```python
from build123d import *

# Parameters (mm, degrees)
F1_DEPTH       = 50.8
F3_DEPTH       = 1066.8
F5_DEPTH       = 26.67
F7_DEPTH       = 76.2
F8_R           = 29.21
F9_DEPTH       = 101.6
F11_DEPTH      = 0.366359725
F13_DEPTH      = 59.2676666667
F14_W          = 33.8666666667
F14_H          = 50.8
F14_W_2        = 25.4
F15_DEPTH      = 25.4
F16_W          = 33.8666666667
F16_H          = 26.3046402751
F16_W_2        = 25.4
F17_DEPTH      = 25.4
F18_R          = 12.7
F19_DEPTH      = 25.4
F19_DEPTH_BACK = 50.8


# Not quite as in the source:
# - a feature names something its author has since deleted; it is built from what else it names


with BuildPart() as f1:
    # F0 (on Top) → F1 (new body)
    with BuildSketch(Plane.XY):
        Polygon((-67.1887439802, 6.1155312845), (282.3736590158, -288.5672921234), (340.6340595151, -239.4534882221), (-8.9283434809, 55.2293351858), (340.6340595151, 349.9121585937), (282.3736590158, 399.025962495), (-67.1887439802, 104.3431390871), (-416.7511469763, 399.025962495), (-475.0115474756, 349.9121585937), (-125.4491444796, 55.2293351858), (-475.0115474756, -239.4534882221), (-416.7511469763, -288.5672921234), align=None)
    extrude(amount=-F1_DEPTH)

    # F2 (on face) → F3 (join)
    with BuildSketch(Plane.XY):
        Polygon((-67.1887439802, 93.3293351858), (-117.9887439802, 55.2293351858), (-67.1887439802, 17.1293351858), (-16.3887439802, 55.2293351858), align=None)
    extrude(amount=F3_DEPTH)

    # F4 (on face) → F5 (cut)
    with BuildSketch(Plane.XY.offset(1066.8)):
        Polygon((-67.1887439802, 17.1293351858), (-33.3220773136, 42.5293351858), (-101.0554106469, 42.5293351858), align=None)
        Polygon((-101.0554106469, 67.9293351858), (-33.3220773136, 67.9293351858), (-67.1887439802, 93.3293351858), align=None)
    extrude(amount=-F5_DEPTH, mode=Mode.SUBTRACT)

    # F6 (on face) → F7 (join)
    with BuildSketch(Plane.XY.offset(1040.13)):
        Polygon((59.8112560198, 93.3293351858), (-67.1887439802, 93.3293351858), (-33.3220773136, 67.9293351858), (-16.3887439802, 55.2293351858), (-33.3220773136, 42.5293351858), (-67.1887439802, 17.1293351858), (59.8112560198, 17.1293351858), align=None)
    extrude(amount=-F7_DEPTH)

    # F8 (on face) → F9 (cut)
    with BuildSketch(Plane.YZ.offset(59.8112560198)):
        with Locations((55.2293351858, 1040.13)):
            Circle(F8_R)
    extrude(amount=-F9_DEPTH, mode=Mode.SUBTRACT)

    # F10 (on face) → F11 (cut, through all)
    with BuildSketch(Plane.XY.offset(1066.8)):
        Polygon((-33.3220773136, 67.9293351858), (-41.7887439802, 67.9293351858), (-41.7887439802, 67.1429912157), (-32.2736186868, 67.1429912157), align=None)
        Polygon((-32.2736186868, 43.3156791558), (-41.7887439802, 43.3156791558), (-41.7887439802, 42.5293351858), (-33.3220773136, 42.5293351858), align=None)
    extrude(amount=-F11_DEPTH, mode=Mode.SUBTRACT)

    # F12 (on face) → F13 (cut, through all)
    with BuildSketch(Plane.YZ.offset(-41.7887439802)):
        with BuildLine():
            Line((42.5293351858, 1040.13), (26.0193351858, 1040.13))
            ThreePointArc((26.0193351858, 1040.13), (30.4887703175, 1024.601685539), (42.5293351858, 1013.8253597249))
            Line((42.5293351858, 1013.8253597249), (42.5293351858, 1040.13))
        make_face()
        with BuildLine():
            Line((84.4393351858, 1040.13), (67.9293351858, 1040.13))
            Line((67.9293351858, 1040.13), (67.9293351858, 1013.8253597249))
            ThreePointArc((67.9293351858, 1013.8253597249), (79.969900054, 1024.601685539), (84.4393351858, 1040.13))
        make_face()
    extrude(amount=-F13_DEPTH, mode=Mode.SUBTRACT)

    # F14 (on face) → F15 (cut)
    with BuildSketch(Plane.XZ.offset(-17.1293351858)):
        with Locations((-84.1220773136, 1014.73)):
            Rectangle(F14_W, F14_H)
        with Locations((-54.4887439802, 1014.73)):
            Rectangle(F14_W_2, F14_H)
    extrude(amount=-F15_DEPTH, mode=Mode.SUBTRACT)

    # F16 (on face) → F17 (cut)
    with BuildSketch(Plane(origin=(0, 93.3293351858, 0), x_dir=(-1, 0, 0), z_dir=(0, 1, 0))):
        with Locations((84.1220773136, 1026.9776798625)):
            Rectangle(F16_W, F16_H)
        with Locations((54.4887439802, 1026.9776798625)):
            Rectangle(F16_W_2, F16_H)
    extrude(amount=-F17_DEPTH, mode=Mode.SUBTRACT)

    # F18 (on face) → F19 (join, two sides)
    with BuildSketch(Plane.XZ.offset(-42.5293351858)) as f19_sk:
        with Locations((-71.4220773136, 1047.75)):
            Circle(F18_R)
    extrude(amount=F19_DEPTH)
    extrude(f19_sk.sketch, amount=-F19_DEPTH_BACK)


solid = f1.part
```
Input: part model. Units: mm. Frame: model coordinates. A direction names the side the tool comes from. Coordinates: 2 decimals unless noted, no trailing zeros. Write each loop counter-clockwise with the first axis right and the second up, starting at its lowest first coordinate (ties: lowest second). Pieces come first, ordered by that corner, then holes.
1) Pin query (flat end, axial travel): pin 1 Ø12.5 at (y, z) = (24.5, 1027.5) entering from -X; pin 2 Ø20.5 at (x, y) = (-68.5, 77) entering from +Z; pin 3 Ø7 at (x, y) = (27, 20) entering from +Z; pin 4 Ø10 at (x, z) = (-122.5, 903.5) entering from +Y. Return the tip coordinate at first contact, or that it passes through.
2) Section C-C on z = 686. Output: boundary loops of the cut face in (x, y).
3) Mould query, pull axis X, two halves, no side actions, for faces 1 (the flat face through (-244.42, -143.29, -25.04)), 2 (the flat face through (-41.43, 74.01, 475.22)), 3 (the flat face through (10, 56, 963.93)). Classes: pulls with the +X half, pulls with the -X half, needs draft (parallel to the pull), parting line crosses it, or undercut.
4) Material intervals for line 1 along Z through (x, y) = (-316, 278.5); line 2 along Y through (x, z) = (-297, -4.5); line 3 along X through (y, z) = (49.5, 880.5), sorted ascending.
5) Set-up query: faces 4 (the cylindrical face through (-74.175, 80.452, 1035.352)), 5 (the flat face through (10, 17.129, 1003)), 6 (the cylindrical face through (-74.175, 30.007, 1035.352)), 7 (the flat face through (-41.789, 86, 1024)). Return all of +Z, -Z, +X, -X, +Y, -Y with unobstructed straight access to the full face (end or side cutting, diameter ignored); none if empty.
6) Section B-B on y = -202. Output: boundary loops of the cut face in (x, z).
7) Section A-A on x = -336. Output: boundary loops of the cut face in (y, z).
Check result:
1. pin 1: stops at x = -41.79
1. pin 2: stops at z = 1066.8
1. pin 3: stops at z = 1040.13
1. pin 4: stops at y = 55.6
2. outline: (-117.99, 55.23) - (-67.19, 17.13) - (-16.39, 55.23) - (-67.19, 93.33) - close
3. face 1: undercut
3. face 2: pulls with the +X half
3. face 3: needs draft
4. line 1: z = -50.8 to 0
4. line 2: y = -187.62 to -89.39, 199.85 to 298.08
4. line 3: x = -110.35 to -24.03
5. face 4: +Y
5. face 5: +Z, +X, -X, -Y
5. face 6: -Y
5. face 7: +Z, +Y
6. outline: (-430.58, -50.8) - (-314.06, -50.8) - (-314.06, 0) - (-430.58, 0) - close; (179.68, -50.8) - (296.21, -50.8) - (296.21, 0) - (179.68, 0) - close
7. outline: (-220.49, -50.8) - (-122.27, -50.8) - (-122.27, 0) - (-220.49, 0) - close; (232.72, -50.8) - (330.95, -50.8) - (330.95, 0) - (232.72, 0) - close
